The listing builds one solid part. Answer for the finished solid, in the listing's coordinates (mm). Face numbers are marked on the shaded views. A direction names the side the tool comes from. Coordinates: 2 decimals unless noted, no trailing zeros. Order: outer loops, then holes, each group sorted by start corner. A loop starts at its lowest first (then second) coordinate and runs counter-clockwise, first axis right, second up. Notation, with made-up numbers: (76, 58.5) -> (128, 58.5) arc R25 ccw to (128, 86.5) -> close; hole circle Ø5 at (-33, 86.5). An arc over 180 degrees is marked (long way). Write item = value, one per line.
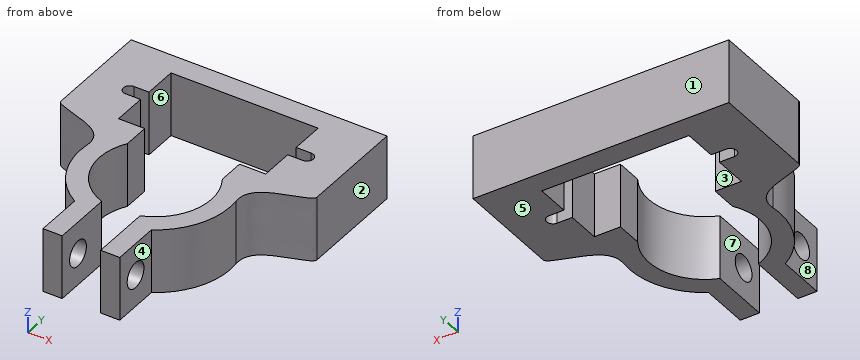
from build123d import *

# Parameters (mm, degrees)
SALIENTE_EXTRUIR1_DEPTH = 10
CROQUIS2_R              = 2
CORTAR_EXTRUIR1_DEPTH   = 27.0000001


with BuildPart() as part:
    # Croquis1 → Saliente-Extruir1 (new body)
    with BuildSketch(Plane.XY):
        with BuildLine():
            Line((11.5, 21.25), (-11.5, 21.25))
            Line((-11.5, 21.25), (-11.5, 16))
            Line((-11.5, 16), (-13.85, 16))
            ThreePointArc((-13.85, 16), (-14.85, 15), (-13.85, 14))
            Line((-13.85, 14), (-11.5, 14))
            Line((-11.5, 14), (-11.5, 8.75))
            Line((-11.5, 8.75), (-7.411101784, 8.75))
            Line((-7.411101784, 8.75), (-7.411101784, 4.65167393))
            ThreePointArc((-7.411101784, 4.65167393), (-8.277405862, -2.836732661), (-3, -8.219641111))
            Line((-3, -8.219641111), (-3, -17.636996672))
            Line((-3, -17.636996672), (-6, -17.636996672))
            Line((-6, -17.636996672), (-6, -10.102598676))
            ThreePointArc((-6, -10.102598676), (-10.54690786, -5.179308313), (-11.662797517, 1.428864608))
            add(Edge.make_bspline(
                [(-20, 8.049530511), (-20, 7.583404659), (-15.923516269, 5.846853582), (-11.193272378, 5.261261744), (-11.662797517, 1.428864608)],
                knots=[0, 0, 0, 0, 0.136185615, 1, 1, 1, 1], degree=3))
            Line((-20, 8.049530511), (-20, 24.696862388))
            Line((-20, 24.696862388), (20, 24.696862388))
            Line((20, 24.696862388), (20, 8.049530511))
            add(Edge.make_bspline(
                [(20, 8.049530511), (20, 7.583404659), (15.923516269, 5.846853582), (11.193272378, 5.261261744), (11.662797517, 1.428864608)],
                knots=[0, 0, 0, 0, 0.136185615, 1, 1, 1, 1], degree=3))
            ThreePointArc((11.662797517, 1.428864608), (10.54690786, -5.179308313), (6, -10.102598676))
            Line((6, -10.102598676), (6, -17.636996672))
            Line((6, -17.636996672), (3, -17.636996672))
            Line((3, -17.636996672), (3, -8.219641111))
            ThreePointArc((3, -8.219641111), (8.277405862, -2.836732661), (7.411101784, 4.65167393))
            Line((7.411101784, 4.65167393), (7.411101784, 8.75))
            Line((7.411101784, 8.75), (11.5, 8.75))
            Line((11.5, 8.75), (11.5, 14))
            Line((11.5, 14), (13.85, 14))
            ThreePointArc((13.85, 14), (14.85, 15), (13.85, 16))
            Line((13.85, 16), (11.5, 16))
            Line((11.5, 16), (11.5, 21.25))
        make_face()
    extrude(amount=SALIENTE_EXTRUIR1_DEPTH)

    # Croquis2 → Cortar-Extruir1 (cut, through all)
    with BuildSketch(Plane.ZY.offset(6)):
        with Locations((5, -13.869797674)):
            Circle(CROQUIS2_R)
    extrude(amount=-CORTAR_EXTRUIR1_DEPTH, mode=Mode.SUBTRACT)


solid = part.part
Q1. The mould has two halves that part along Y. Classify the marked faces 1, 2 and 3: released by +Y, released by -Y, zero draft, split by the parting line, or undercut.
The answers:
face_1 = released by +Y
face_2 = zero draft
face_3 = undercut
Q2. Section D-D, the plane z = 4.5 is taken. Give the number of separate pieces and of enclosed holes in the cut face, plus the area to 3 significant figures.
The answers:
separate_pieces = 3
enclosed_holes = 0
area = 547 mm2
Q3. A tool of negligible diameter and unlimited length cuts with its end or side. For the marked faces 4, 5, 6, 7 and 8, from which of +Z, -Z, +X, -X, +Y, -Y can it reach the whole face along a straight path? Write none if from no direction.
The answers:
face_4 = +Z, -Z, +X, -Y
face_5 = -Z, +X, -X, +Y, -Y
face_6 = +Z, -Z
face_7 = +Z, -Z, -Y
face_8 = +Z, -Z, -X, -Y
Q4. Section B-B, the plane x = 10 is taken. Give the vertices of the cut face in (y, z).
The answers:
outline = (-6.17, 0) -> (8.75, 0) -> (8.75, 10) -> (-6.17, 10) -> close; (21.25, 0) -> (24.7, 0) -> (24.7, 10) -> (21.25, 10) -> close
Q5. Section A-A, the plane y = 15 is taken. Give the vertices of the cut face in (x, z).
The answers:
outline = (-20, 0) -> (-14.85, 0) -> (-14.85, 10) -> (-20, 10) -> close; (14.85, 0) -> (20, 0) -> (20, 10) -> (14.85, 10) -> close
Q6. Find the intervals of material crossed by line 1 along Y through (x, z) = (4.65, 5); line 2 along X through (y, z) = (12, 1.75); line 3 along X through (y, z) = (-15.5, 8), in increasing order.
The answers:
line_1 = -17.64 to -15.87, -11.87 to -7.41, 21.25 to 24.7
line_2 = -20 to -11.5, 11.5 to 20
line_3 = -6 to -3, 3 to 6
Q7. Section C-C, the plane x = 1 is taken. Give the vertices of the cut face in (y, z).
The answers:
outline = (21.25, 0) -> (24.7, 0) -> (24.7, 10) -> (21.25, 10) -> close
Q8. Each of these flat-tipped pins is pushed along its axis until it touches: pin 1 Ø1.5 at (y, z) = (-9.5, 9) entering from -X; pin 2 Ø1.2 at (y, z) = (7, 7) entering from -X. Where does it stop, or does it pass through?
The answers:
pin_1 = -7.84
pin_2 = -19.78
